Geometry: final body of the model. Coordinates: model frame, mm. Face numbers are marked on the shaded views. A direction names the side the tool comes from. Give positions to 0.01 mm unless a question says otherwise; leave off trailing zeros. Write each loop counter-clockwise with the first axis right and the second up, starting at its lowest first coordinate (ties: lowest second). Pieces come first, ordered by that corner, then holes. Notation, with made-up numbers: M 59.25,87.25 L 78.25,87.25 A9 ccw 78.25,102.25 Z; hole C -40,-40 d8. An arc over 180 degrees is marked long. Use a Markdown table: item, result. Add a question column.
1) Pin query (flat end, axial travel): pin 1 (5 mm diameter, centred on y = 77, z = 0.5, fed in from +X); pin 2 (4 mm diameter, centred on y = 57, z = 4.5, fed in from -X); pin 3 (1.5 mm diameter, centred on x = 2, y = 52, fed in from +Z); pin 4 (5 mm diameter, centred on x = 4.5, y = 23, fed in from -Z). Return the tip coordinate at first contact, or that it passes through.
2) Section D-D on y = 58. Return the cut outline in (x, z).
3) Set-up query: the marked faces 1 and 2. Return all of +Z, -Z, +X, -X, +Y, -Y with unobstructed straight access to the full face (end or side cutting, diameter ignored); none if empty.
4) Draft query along X for the marked faces 3, 4 and 5. Return one class per face: +X half, -X half, draft (parallel to the pull), parting line (faces both ways), or undercut.
5) Line query: line 1 (Y direction, x = -2.75, z = -4); line 2 (X direction, y = 12, z = 0.25); line 3 (Y direction, x = 1.5, z = -0.25). Output: solid intervals per line, ascending.
6) Section C-C on x = 0. Return the cut outline in (y, z).
7) Section B-B on z = 0. State how many separate pieces and enclosed holes the cut face has, then the cut area to 3 significant figures.
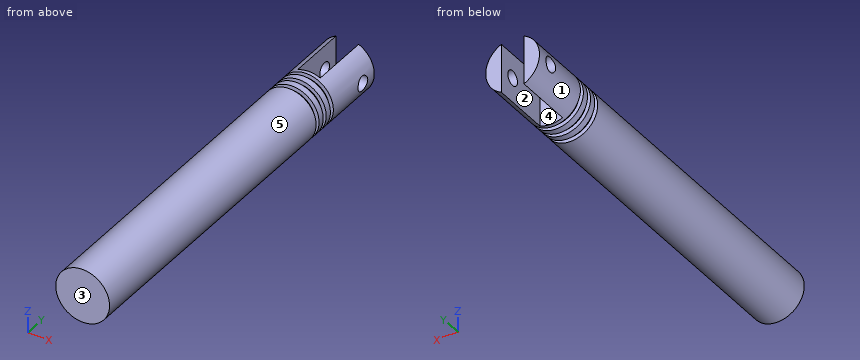
```python
from build123d import *

# Parameters (mm, degrees)
SKETCH1_R               = 5.56895
BOSS_EXTRUDE1_DEPTH     = 84.66582
SKETCH2_W               = 4.699
SKETCH2_H               = 16.131480258
CUT_EXTRUDE1_DEPTH      = 12.319
CUT_EXTRUDE2_DEPTH      = 86.031332369
CUT_EXTRUDE2_DEPTH_BACK = 86.031332369
SKETCH3_R               = 1.5494
SKETCH4_W               = 0.843885596
SKETCH4_H               = 0.947610215
LPATTERN1_COUNT         = 3
LPATTERN1_PITCH         = 2.286


with BuildPart() as part:
    # Sketch1 → Boss-Extrude1 (new body)
    with BuildSketch(Plane(origin=(0, 0, 0), x_dir=(1, 0, 0), z_dir=(0, 1, 0))):
        with Locations(Location((0, 0, 0), (0, 0, 270))):
            Circle(SKETCH1_R)
    extrude(amount=BOSS_EXTRUDE1_DEPTH)

    # Sketch2 → Cut-Extrude1 (cut)
    with BuildSketch(Plane(origin=(0, 84.66582, 0), x_dir=(1, 0, 0), z_dir=(0, 1, 0))):
        Rectangle(SKETCH2_W, SKETCH2_H)
    extrude(amount=-CUT_EXTRUDE1_DEPTH, mode=Mode.SUBTRACT)

    # Sketch3 → Cut-Extrude2 (cut, two sides: drawn at the far end of the back side and taken through both)
    with BuildSketch(Plane(origin=(0, 0, 0), x_dir=(0, 0, -1), z_dir=(1, 0, 0)).offset(-CUT_EXTRUDE2_DEPTH_BACK)):
        with Locations(Location((0, 81.03362, 0), (0, 0, 270))):
            Circle(SKETCH3_R)
    extrude(amount=CUT_EXTRUDE2_DEPTH + CUT_EXTRUDE2_DEPTH_BACK, mode=Mode.SUBTRACT)

    # Sketch4 → Cut-Revolve1 (revolve, cut)
    with BuildSketch(Plane(origin=(0, 0, 0), x_dir=(0, 0, -1), z_dir=(1, 0, 0))):
        with Locations((5.147007202, 71.109959008)):
            Rectangle(SKETCH4_W, SKETCH4_H)
    cut_revolve1 = revolve(axis=Axis((0, -4.233291, 0), (0, 1, 0)), mode=Mode.SUBTRACT)

    # LPattern1: Cut-Revolve1 ×3
    with Locations(*[(0, -i * LPATTERN1_PITCH, 0) for i in range(1, LPATTERN1_COUNT)]):
        add(cut_revolve1, mode=Mode.SUBTRACT)


solid = part.part
```
Found:
| question | item | result |
|---|---|---|
| 1 | pin 1 | x = 5.57 |
| 1 | pin 2 | x = -4.98 |
| 1 | pin 3 | z = 5.43 |
| 1 | pin 4 | z = -5.2 |
| 2 | outline | C 0,0 d11.14 |
| 3 | face 1 | +Y, -Y |
| 3 | face 2 | +Z, -Z, +Y |
| 4 | face 3 | draft |
| 4 | face 4 | undercut |
| 4 | face 5 | parting line |
| 5 | line 1 | 0 to 66.06, 67.01 to 68.35, 69.3 to 70.64, 71.58 to 84.67 |
| 5 | line 2 | -5.56 to 5.56 |
| 5 | line 3 | 0 to 72.35 |
| 6 | outline | M 0,-5.57 L 66.06,-5.57 L 66.06,-4.73 L 67.01,-4.73 L 67.01,-5.57 L 68.35,-5.57 L 68.35,-4.73 L 69.3,-4.73 L 69.3,-5.57 L 70.64,-5.57 L 70.64,-4.73 L 71.58,-4.73 L 71.58,-5.57 L 72.35,-5.57 L 72.35,5.57 L 71.58,5.57 L 71.58,4.73 L 70.64,4.73 L 70.64,5.57 L 69.3,5.57 L 69.3,4.73 L 68.35,4.73 L 68.35,5.57 L 67.01,5.57 L 67.01,4.73 L 66.06,4.73 L 66.06,5.57 L 0,5.57 Z |
| 7 | separate pieces | 3 |
| 7 | enclosed holes | 0 |
| 7 | area | 860 mm² |
